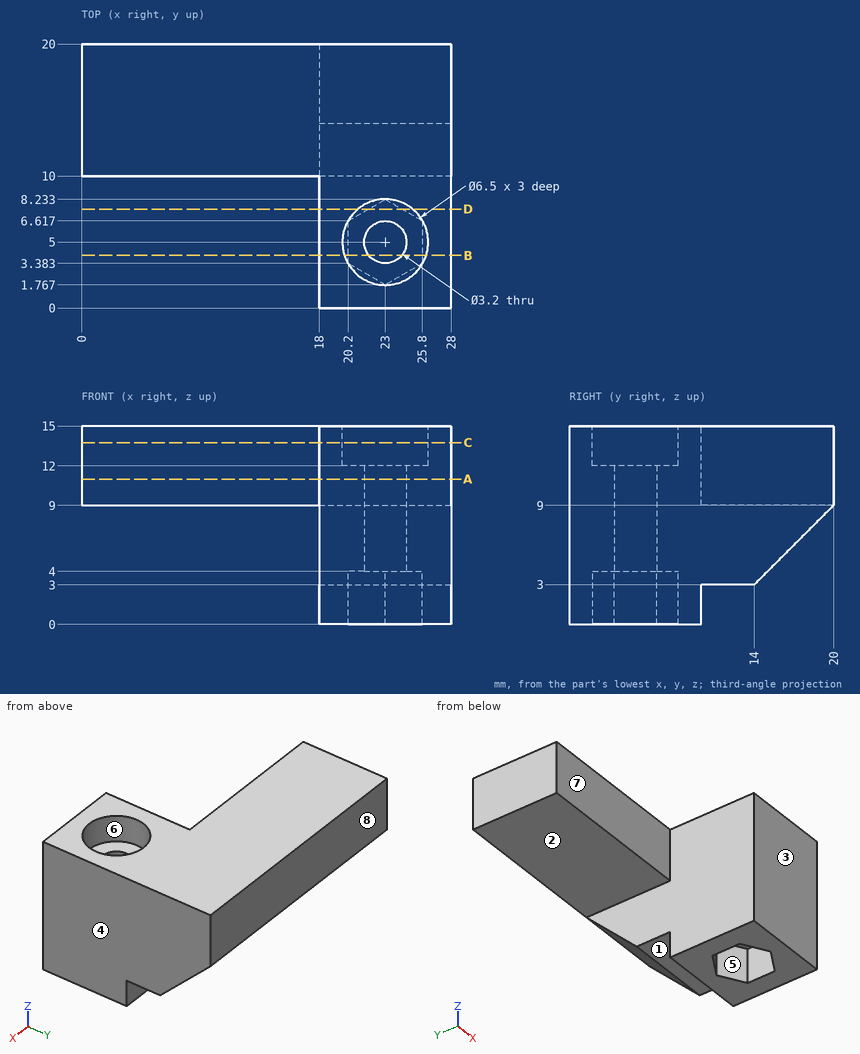
Answer from the drawing. Dimensions are ordinates in mm from the lowest x, y and z of the part. A direction names the side the tool comes from. Give positions to 0.01 mm unless a question says otherwise; leave off trailing zeros. Loops run counter-clockwise (first coordinate to the right, second up) from the corner with the lowest first, then second, coordinate; pieces in that order, holes last. Notation, with made-up numbers: M 38.5,-27 L 65.5,-27 A33 cw 65.5,10 Z; hole C 46,-21 d3. An arc over 180 degrees is marked long. One line per item, written item: value.
Q1. Flat-ended cylindrical pins translate along their axes: P1, Ø3, axis at x = 11, z = 13, coming from the -Y side; P2, Ø3.5, axis at y = 4.5, z = 1.5, coming from the -X side; P3, Ø8, axis at x = 7.5, y = 16, coming from the -Z side. Find the tip coordinate at first contact, or state that the pin passes through.
Working result:
P1: stops at y = 10
P2: stops at x = 18
P3: stops at z = 9
Q2. A cutting plane is placed at A-A on z = 11. Determine the outline of the cut face in (x, y).
Working result:
outline: M 0,10 L 18,10 L 18,0 L 28,0 L 28,20 L 0,20 Z; hole C 23,5 d3.2
Q3. A cutting plane is placed at C-C on z = 13.75. Determine the outline of the cut face in (x, y), then the cut area to 3 significant figures.
Working result:
outline: M 0,10 L 18,10 L 18,0 L 28,0 L 28,20 L 0,20 Z; hole C 23,5 d6.5
area: 347 mm^2
Q4. Determine the mould class of the marked faces 6, 7 and 8 for opening direction Y: +Y half, -Y half, draft (parallel to the pull), parting line (faces both ways), or undercut.
Working result:
face 6: undercut
face 7: -Y half
face 8: +Y half
Q5. A cutting plane is placed at D-D on y = 7.5. Determine the outline of the cut face in (x, z), then the cut area to 3 significant figures.
Working result:
outline: M 18,0 L 21.73,0 L 21.73,4 L 24.27,4 L 24.27,0 L 28,0 L 28,15 L 25.08,15 L 25.08,12 L 20.92,12 L 20.92,15 L 18,15 Z
area: 127 mm^2
Q6. A cutting plane is placed at B-B on y = 4. Determine the outline of the cut face in (x, z).
Working result:
outline: M 18,0 L 20.2,0 L 20.2,4 L 21.75,4 L 21.75,12 L 19.91,12 L 19.91,15 L 18,15 Z; M 24.25,4 L 25.8,4 L 25.8,0 L 28,0 L 28,15 L 26.09,15 L 26.09,12 L 24.25,12 Z
Q7. Find the intervals of material crossed by line 1 (Y direction, x = 23, z = 9); line 2 (Y direction, x = 23, z = 13.35); line 3 (X direction, y = 9.75, z = 10), in increasing order. Write a range as from..to.
Working result:
line 1: y = 0..3.4, 6.6..20
line 2: y = 0..1.75, 8.25..20
line 3: x = 18..28
Q8. For the marked faces 1, 2, 3, 4 and 5, determine the directions among +Z, -Z, +X, -X, +Y, -Y from which every point of the face is accessible in a straight line to the end or side of a thin tool.
Working result:
face 1: -Z, +X, -X, +Y
face 2: -Z, -X, +Y, -Y
face 3: +Z, -Z, +X, -X, -Y
face 4: +Z, -Z, +X, +Y, -Y
face 5: -Z
